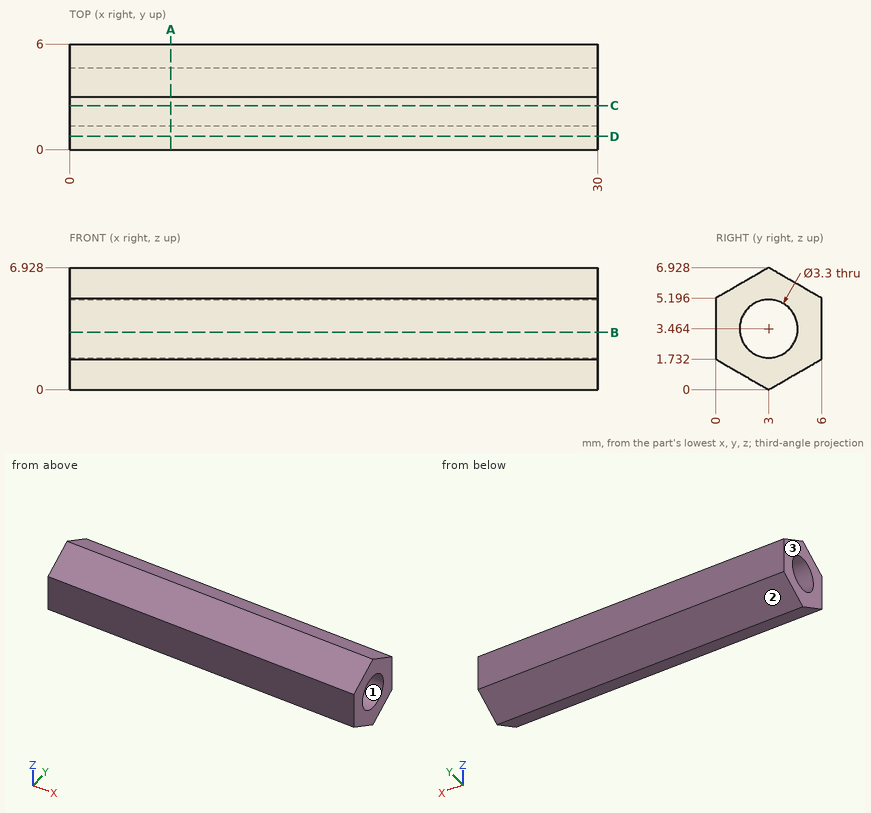
Source: three-view drawing plus pictorial views. Frame: mm from the lowest corner of the part. Coordinates: 2 decimals unless noted, no trailing zeros. Write each loop counter-clockwise with the first axis right and the second up, starting at its lowest first coordinate (ties: lowest second). Pieces come first, ordered by that corner, then holes. Notation, with made-up numbers: (14.5, -25) -> (43.5, -25) arc R22 cw to (43.5, -11) -> close; hole circle Ø1 at (42, 26). An arc over 180 degrees is marked (long way). Answer as a JSON object with one key per item and string values.
1. Section D-D on y = 0.75. Return the cut outline in (x, z).
Result set:
{"outline": "(0, 1.3) -> (30, 1.3) -> (30, 5.63) -> (0, 5.63) -> close"}
2. Section C-C on y = 2.5. Return the cut outline in (x, z).
Result set:
{"outline": "(0, 0.29) -> (30, 0.29) -> (30, 1.89) -> (0, 1.89) -> close; (0, 5.04) -> (30, 5.04) -> (30, 6.64) -> (0, 6.64) -> close"}
3. Material intervals for line 1 (Y direction, x = 19, z = 3.5); line 2 (Y direction, x = 8.75, z = 4.5) (1 decimal); line 3 (Z direction, x = 21.75, y = 4), sorted ascending. Write a range as from..to.
Result set:
{"line 1": "y = 0..1.35, 4.65..6", "line 2": "y = 0..1.7, 4.3..6", "line 3": "z = 0.58..2.15, 4.78..6.35"}
4. First-contact query: P1, Ø1, axis at y = 3.5, z = 3, coming from the +X side; P2, Ø1.5, axis at x = 16.5, z = 6, coming from the -Y side; P3, Ø1.5, axis at y = 2.5, z = 4.5, coming from the -X side. Flat tips, straight axial feed; report the tip coordinate or a pass-through.
Result set:
{"P1": "passes through", "P2": "stops at y = 0.09", "P3": "stops at x = 0"}
5. Section A-A on x = 5.75. Return the cut outline in (y, z).
Result set:
{"outline": "(0, 1.73) -> (3, 0) -> (6, 1.73) -> (6, 5.2) -> (3, 6.93) -> (0, 5.2) -> close; hole circle Ø3.3 at (3, 3.46)"}
6. Section B-B on z = 3.25. Return the cut outline in (x, y).
Result set:
{"outline": "(0, 0) -> (30, 0) -> (30, 1.36) -> (0, 1.36) -> close; (0, 4.64) -> (30, 4.64) -> (30, 6) -> (0, 6) -> close"}
7. Mould query, pull axis Z, two halves, no side actions, for the marked faces 1, 2 and 3. Classes: released by +Z, released by -Z, zero draft, split by the parting line, or undercut.
Result set:
{"face 1": "undercut", "face 2": "released by -Z", "face 3": "zero draft"}
